```python
from build123d import *

# Parameters (mm, degrees)
CROQUIS1_R              = 4
SALIENTE_EXTRUIR1_DEPTH = 37.05
SALIENTE_EXTRUIR2_DEPTH = 22
REDONDEO1_R             = 0.5
REDONDEO2_R             = 1
CROQUIS3_R              = 1.1
CORTAR_EXTRUIR1_DEPTH   = 20


with BuildPart() as part:
    # Croquis1 → Saliente-Extruir1 (new body)
    with BuildSketch(Plane(origin=(0, 0, 0), x_dir=(0, 0, -1), z_dir=(1, 0, 0))):
        Circle(CROQUIS1_R)
    extrude(amount=SALIENTE_EXTRUIR1_DEPTH)

    # Croquis2 → Saliente-Extruir2 (add)
    with BuildSketch(Plane(origin=(37.05, 0, 0), x_dir=(0, 0, -1), z_dir=(1, 0, 0))):
        Polygon((0, -8.544783984), (7.4, -4.272391992), (7.4, 4.272391992), (0, 8.544783984), (-7.4, 4.272391992), (-7.4, -4.272391992), align=None)
    extrude(amount=SALIENTE_EXTRUIR2_DEPTH)

    # Redondeo1
    redondeo1_edges = [part.edges().sort_by_distance(p)[0] for p in [
        (37.05, 0, 4),
        (37.05, -6.408587988, 3.7),
        (37.05, -6.408587988, -3.7),
        (37.05, 0, -7.4),
        (37.05, 6.408587988, -3.7),
        (37.05, 6.408587988, 3.7),
        (37.05, 0, 7.4),
        (59.05, -6.408587988, 3.7),
        (59.05, -6.408587988, -3.7),
        (59.05, 0, -7.4),
        (59.05, 6.408587988, -3.7),
        (59.05, 6.408587988, 3.7),
        (59.05, 0, 7.4),
    ]]
    fillet(redondeo1_edges, radius=REDONDEO1_R)

    # Redondeo2
    redondeo2_edges = [part.edges().sort_by_distance(p)[0] for p in [
        (0, 0, 4),
    ]]
    fillet(redondeo2_edges, radius=REDONDEO2_R)

    # Croquis3 → Cortar-Extruir1 (cut)
    with BuildSketch(Plane(origin=(0, 6.408587988, -3.7), x_dir=(1, 0, 0), z_dir=(0, 0.8660254037844386, -0.5000000000000003))):
        with Locations(Location((44.925, 0, 0), (0, 0, 270))):
            Circle(CROQUIS3_R)
    extrude(amount=-CORTAR_EXTRUIR1_DEPTH, mode=Mode.SUBTRACT)


solid = part.part
```
Design review of the part built by this model. Coordinates are the model's own, in mm. A direction names the side the tool comes from. Give positions to 0.01 mm unless a question says otherwise; leave off trailing zeros. Order: outer loops, then holes, each group sorted by start corner. A loop starts at its lowest first (then second) coordinate and runs counter-clockwise, first axis right, second up. Notation, with made-up numbers: (-6.5, -33) -> (39.5, -33) arc R32 ccw to (39.5, 4) -> close; hole circle Ø6 at (-32.75, -23). An arc over 180 degrees is marked (long way). Write item = value, one per line. Start each with the question number.
(1) We need section C-C on x = 8. Write out the cut boundary in (y, z), plus the area to 3 significant figures.
(2) For pin 1 (1.5 mm diameter, centred on x = 13, y = 3, fed in from +Z); pin 2 (5 mm diameter, centred on y = 5.5, z = -4.5, fed in from -X); pin 3 (1 mm diameter, centred on x = 13.5, z = -4, fed in from +Y), all flat-tipped, find the tip position at first contact; note any pin that passes through.
(3) We need section A-A on x = 45.5. Write out the cut boundary in (y, z).
(4) For faces 4 (the face through (18.526, -3.905, 0.867)), 5 (the face through (58.9, -6.3, 3.6)), list the 3-axis set-ups (+Z, -Z, +X, -X, +Y, -Y) from which the entire face can be reached by the end or side of a thin tool; tool diameter is ignored.
(5) Mouldability with a two-part tool opening along X and no side actions: class faces 1 (the face through (43.85, -0.03, -0.26)), 2 (the face through (58.9, 6.3, -3.6)), 3 (the face through (47.903, -6.438, -3.648)) as +X half, -X half, draft (parallel to the pull), parting line (faces both ways), or undercut.
(6) To check wall thickness, follow line 1 along X through (y, z) = (2.75, -0.5); line 2 along X through (y, z) = (-3.25, 4); line 3 along Y through (x, z) = (49, 1). State the ranges of each line that lie inside material, in increasing order.
(7) We need section B-B on x = 38.5. Write out the cut boundary in (y, z), plus the area to 3 significant figures.
Numbers:
q1.outline = circle Ø8 at (0, 0)
q1.area = 50.3 mm^2
q2.pin_1 = 3.31
q2.pin_2 = 37.05
q2.pin_3 = 1.94
q3.outline = (-8.54, 0) -> (-4.27, -7.4) -> (4.27, -7.4) -> (5.94, -4.51) -> (-6.88, 2.89) -> close; (-5.94, 4.51) -> (6.88, -2.89) -> (8.54, 0) -> (4.27, 7.4) -> (-4.27, 7.4) -> close
q4.face_4 = -X
q4.face_5 = +Z, +X, -Y
q5.face_1 = undercut
q5.face_2 = +X half
q5.face_3 = draft
q6.line_1 = 0 to 44.36, 45.49 to 59.05
q6.line_2 = 37.05 to 59.05
q6.line_3 = -7.97 to 7.97
q7.outline = (-8.54, 0) -> (-4.27, -7.4) -> (4.27, -7.4) -> (8.54, 0) -> (4.27, 7.4) -> (-4.27, 7.4) -> close
q7.area = 190 mm^2
